Autodesk Inventor part; units mm, degrees
ref_plane "YZ Plane" through (0, 0, 0) normal (1, 0, 0) x (0, 1, 0)
ref_plane "XZ Plane" through (0, 0, 0) normal (0, 1, 0) x (-1, 0, 0)
ref_plane "XY Plane" through (0, 0, 0) normal (0, 0, 1) x (1, 0, 0)
sketch "Sketch1" plane through (0, 0, 0) normal (0, 0, 1) x (1, 0, 0)
  circle A0 centre (0, 0) radius 2.9845
  circle A1 centre (0, 0) radius 5.842
  circle A2 centre (0, 0) radius 3.302
  dimension "d0" = 5.969
  dimension "d2" = 0.3175
  dimension "d5" = 2.54
extrude "Extrusion1" add sketch "Sketch1" along normal blind 25.4 contours A1
sketch "Sketch2" plane through (0, 0, 25.4) normal (0, 0, 1) x (1, 0, 0)
  circle A0 centre (0, 0) radius 5.842
extrude "Extrusion2" add sketch "Sketch2" along normal blind 3.175
sketch "Sketch3" plane through (0, 0, 28.575) normal (0, 0, 1) x (1, 0, 0)
  line L0 (0.635, -2.54) -> (-0.635, -2.54)
  line L1 (-0.635, -2.54) -> (-0.635, 2.54)
  line L2 (-0.635, 2.54) -> (0.635, 2.54)
  line L3 (0.635, 2.54) -> (0.635, -2.54)
  line L4 (0.635, -2.54) -> (-0.635, 2.54) construction
  line L5 (-0.635, -2.54) -> (0.635, 2.54) construction
  line L6 (0, 2.54) -> (0, -2.54) construction
  line L7 (-1.905, 2.54) -> (1.905, 2.54)
  line L8 (1.905, 2.54) -> (0, 5.08)
  line L9 (0, 5.08) -> (-1.905, 2.54)
  point P0 (0, 0)
  dimension "d8" = 5.08
  dimension "d9" = 2.54
  dimension "d10" = 1.27
  dimension "d11" = 3.81
extrude "Extrusion3" cut sketch "Sketch3" against normal blind 1.27
chamfer "Chamfer1" distance 0.508 angle 45 1 edges at (-5.842, 0, 28.575)
sketch "Sketch6" plane through (0, 0, 25.4) normal (0, 0, -1) x (-1, 0, 0)
  circle A0 centre (0, 0) radius 3.302
  line L0 (0.6206, 3.2432) -> (3.1189, -1.0842) construction
  line L1 (3.1189, 1.0842) -> (0.6206, -3.2432)
  line L2 (0, 0) -> (3.302, 0) construction
  circle A1 centre (0, 0) radius 3.302 construction
  line L3 (0, 0) -> (2.8596, -1.651) construction
  line L4 (0, 0) -> (2.8596, 1.651) construction
  line L5 (-1.3144, 4.3273) -> (-3.8128, 0) construction
  arc A2 (0.6206, -3.2432) -> (3.1189, 1.0842) centre (0, 0) ccw
  dimension "d24" = 60
  dimension "d26" = 5.461
extrude "Extrusion6" add sketch "Sketch6" along normal blind 10.16 contours A0 L1 picked at (1.6947, -1.725)
sketch "Sketch7" plane through (0, 0, 28.575) normal (0, 0, 1) x (1, 0, 0)
  circle A0 centre (0, 0) radius 5.842
extrude "Extrusion7" cut sketch "Sketch7" against normal blind 6.35 keep common part
equation "\"d9\" = 0.5 * d8"
equation "\"d11\" = 3 * d10"
properties part number "testpotcap"
Could you check a few things on this model? Use its own coordinates, in mm. A direction names the side the tool comes from. Round coordinates to 2 decimals unless told otherwise and drop trailing zeros. Loops run counter-clockwise (first coordinate to the right, second up) from the corner with the lowest first, then second, coordinate; pieces in that order, holes last.
Q1. For P1, Ø1, axis at x = 1.5, z = 27.5, coming from the +Y side; P2, Ø1, axis at y = -2, z = 23, coming from the -X side, each with a flat end and sliding along its axis, tell me the tip position at first contact or that it passes through.
Q2. On a 3-axis mill with a long thin cutter (end or side, diameter ignored), from which of +Z, -Z, +X, -X, +Y, -Y can I reach the whole of each face in a straight line? I mean faces 4 (the flat face through (0.635, 0, 28)), 5 (the flat face through (1, 0, 28.575)), 6 (the cylindrical face through (2.805, 1.742, 23.79)). Say none if no direction works.
Q3. I want a section at B-B (y = 0). Write out the boundary of the cut face in (x, z) (3 decimals), and give its area (3 significant figures).
Q4. Please list where these lines run through material, in increasing order: L1, parallel to Y at x = 0, z = 23.1; L2, parallel to Z at x = -0.5, y = 1.25 (3 decimals); L3, parallel to Y at x = 2, z = 24.5.
Q5. I want a section at A-A (z = 25.75). Write out the boundary of the cut face in (x, y), and give its area (3 significant figures).
Q6. Thinking about a two-plate mould opening in Y: for faces 1 (the flat face through (-0.94, 3.83, 27.95)), 2 (the cylindrical face through (-1.266, 5.703, 25.105)), 3 (the flat face through (-1, -3, 22.225)), which applies, pulls with the +Y half, pulls with the -Y half, needs draft (parallel to the pull), parting line crosses it, or undercut?
Answer below:
1. P1: stops at y = 5.76
1. P2: stops at x = -5.65
2. face 4: +Z
2. face 5: +Z, +X, -X, +Y, -Y
2. face 6: -Z
3. outline: (-5.842, 22.225) - (-2.493, 22.225) - (-2.493, 25.4) - (3.302, 25.4) - (3.302, 22.225) - (5.842, 22.225) - (5.842, 28.067) - (5.334, 28.575) - (0.635, 28.575) - (0.635, 27.305) - (-0.635, 27.305) - (-0.635, 28.575) - (-5.334, 28.575) - (-5.842, 28.067) - close
3. area: 53.9 mm2
4. L1: y = -5.84 to -3.3, 3.3 to 5.84
4. L2: z = 25.4 to 27.305
4. L3: y = -5.49 to -2.63, 2.63 to 5.49
5. outline: circle Ø11.68 at (0, 0)
5. area: 107 mm2
6. face 1: undercut
6. face 2: parting line crosses it
6. face 3: needs draft
